```python
from build123d import *

# Parameters (mm, degrees)
F0_R     = 0.4
F0_W     = 3.627236
F0_H     = 6.562536
F0_W_2   = 7.74
F0_H_2   = 7.54
F0_W_3   = 1.741074
F0_H_3   = 3.515658
F1_DEPTH = 0.8
F2_W     = 1.5
F2_H     = 7.54
F2_W_2   = 7.74
F3_DEPTH = 3.7
F4_DEPTH = 0.6
F2_W_3   = 3.627236
F2_H_2   = 6.562536
F2_W_4   = 1.741074
F2_H_3   = 3.515658
F5_DEPTH = 1.8
F6_DEPTH = 2.5
F7_W     = 3.138918
F7_H     = 1.686543
F7_W_2   = 7.430458
F7_H_2   = 3.743672
F7_W_3   = 2.755912
F7_H_3   = 4.345508
F7_W_4   = 2.256349
F7_H_4   = 1.289181
F8_DEPTH = 1.5


with BuildPart() as f1:
    # F0 (on Top) → F1 (new body, symmetric)
    with BuildSketch(Plane.XY):
        Polygon((21.675, -8.905), (21.675, 8.905), (-21.675, 8.905), (-21.675, 3.77), (-13.935, 3.77), (-13.935, -3.77), (-21.675, -3.77), (-21.675, -8.905), align=None)
        with Locations((-19.378522, -6.999998)):
            Circle(F0_R, mode=Mode.SUBTRACT)
        with Locations((-16.578532, -6.992826)):
            Circle(F0_R, mode=Mode.SUBTRACT)
        with Locations((-13.778541, -6.985653)):
            Circle(F0_R, mode=Mode.SUBTRACT)
        with Locations((-10.97855, -6.978481)):
            Circle(F0_R, mode=Mode.SUBTRACT)
        with Locations((-8.178559, -6.971308)):
            Circle(F0_R, mode=Mode.SUBTRACT)
        with Locations((-5.378568, -6.964136)):
            Circle(F0_R, mode=Mode.SUBTRACT)
        with Locations((-2.578578, -6.956963)):
            Circle(F0_R, mode=Mode.SUBTRACT)
        with Locations((0.221413, -6.949791)):
            Circle(F0_R, mode=Mode.SUBTRACT)
        with Locations((3.021404, -6.942618)):
            Circle(F0_R, mode=Mode.SUBTRACT)
        with Locations((5.821395, -6.935446)):
            Circle(F0_R, mode=Mode.SUBTRACT)
        with Locations((8.621386, -6.928273)):
            Circle(F0_R, mode=Mode.SUBTRACT)
        with Locations((11.421377, -6.921101)):
            Circle(F0_R, mode=Mode.SUBTRACT)
        with Locations((14.221367, -6.913928)):
            Circle(F0_R, mode=Mode.SUBTRACT)
        with Locations((17.021358, -6.906755)):
            Circle(F0_R, mode=Mode.SUBTRACT)
        with Locations((19.821349, -6.899583)):
            Circle(F0_R, mode=Mode.SUBTRACT)
        Polygon((-0.115967, -0.994175), (-5.560689, -6.438898), (-11.005411, -0.994175), (-5.560689, 4.450547), align=None, mode=Mode.SUBTRACT)
        with Locations((16.957284, -2.671687)):
            Circle(F0_R, mode=Mode.SUBTRACT)
        with Locations((19.757274, -2.664514)):
            Circle(F0_R, mode=Mode.SUBTRACT)
        with Locations((16.978642, -0.005869)):
            Circle(F0_R, mode=Mode.SUBTRACT)
        with Locations((5.141591, 0)):
            Rectangle(F0_W, F0_H, mode=Mode.SUBTRACT)
        with Locations((19.778633, 0.001303)):
            Circle(F0_R, mode=Mode.SUBTRACT)
        with Locations((17, 2.659948)):
            Circle(F0_R, mode=Mode.SUBTRACT)
        with Locations((19.799991, 2.667121)):
            Circle(F0_R, mode=Mode.SUBTRACT)
        with Locations((-19.378522, 7.092626)):
            Circle(F0_R, mode=Mode.SUBTRACT)
        with Locations((-16.578532, 7.099799)):
            Circle(F0_R, mode=Mode.SUBTRACT)
        with Locations((-13.778541, 7.106971)):
            Circle(F0_R, mode=Mode.SUBTRACT)
        with Locations((-10.97855, 7.114144)):
            Circle(F0_R, mode=Mode.SUBTRACT)
        with Locations((-8.178559, 7.121316)):
            Circle(F0_R, mode=Mode.SUBTRACT)
        with Locations((-5.378568, 7.128489)):
            Circle(F0_R, mode=Mode.SUBTRACT)
        with Locations((-2.578578, 7.135661)):
            Circle(F0_R, mode=Mode.SUBTRACT)
        with Locations((0.221413, 7.142834)):
            Circle(F0_R, mode=Mode.SUBTRACT)
        with Locations((3.021404, 7.150007)):
            Circle(F0_R, mode=Mode.SUBTRACT)
        with Locations((5.821395, 7.157179)):
            Circle(F0_R, mode=Mode.SUBTRACT)
        with Locations((8.621386, 7.164352)):
            Circle(F0_R, mode=Mode.SUBTRACT)
        with Locations((11.421377, 7.171524)):
            Circle(F0_R, mode=Mode.SUBTRACT)
        with Locations((14.221367, 7.178697)):
            Circle(F0_R, mode=Mode.SUBTRACT)
        with Locations((17.021358, 7.185869)):
            Circle(F0_R, mode=Mode.SUBTRACT)
        with Locations((19.821349, 7.193042)):
            Circle(F0_R, mode=Mode.SUBTRACT)
        with Locations((-17.805, 0)):
            Rectangle(F0_W_2, F0_H_2)
        Polygon((-11.005411, -0.994175), (-5.560689, -6.438898), (-0.115967, -0.994175), (-5.560689, 4.450547), align=None)
        with Locations((5.141591, 0)):
            Rectangle(F0_W, F0_H)
        with Locations((5.141591, 0)):
            Rectangle(F0_W_3, F0_H_3, mode=Mode.SUBTRACT)
        with Locations((5.141591, 0)):
            Rectangle(F0_W_3, F0_H_3)
    extrude(amount=F1_DEPTH, both=True)

    # F2 (on face) → F3 (join)
    with BuildSketch(Plane.XY.offset(0.8)):
        with Locations((-22.425, 0)):
            Rectangle(F2_W, F2_H)
        with Locations((-17.805, 0)):
            Rectangle(F2_W_2, F2_H)
    extrude(amount=F3_DEPTH)

    # F2 (on face) → F4 (join)
    with BuildSketch(Plane.XY.offset(0.8)):
        Polygon((-5.560689, 5.444722), (-11.005411, 0), (-5.560689, -5.538898), (0, 0), align=None)
    extrude(amount=F4_DEPTH)

    # F2 (on face) → F5 (join)
    with BuildSketch(Plane.XY.offset(0.8)):
        with Locations((5.141591, 0)):
            Rectangle(F2_W_3, F2_H_2)
        with Locations((5.141591, 0)):
            Rectangle(F2_W_4, F2_H_3, mode=Mode.SUBTRACT)
    extrude(amount=F5_DEPTH)

    # F2 (on face) → F6 (join)
    with BuildSketch(Plane.XY.offset(0.8)):
        with Locations((5.141591, 0)):
            Rectangle(F2_W_4, F2_H_3)
    extrude(amount=F6_DEPTH)

    # F7 (on face) → F8 (join)
    with BuildSketch(Plane(origin=(0, 0, -0.8), x_dir=(1, 0, 0), z_dir=(0, 0, -1))):
        with Locations((-19.302629, -5.330686)):
            Rectangle(F7_W, F7_H)
        with Locations((-12.91917, 0)):
            Rectangle(F7_W_2, F7_H_2)
        with Locations((12.990596, 3.507671)):
            Rectangle(F7_W_3, F7_H_3)
        with Locations((13.02365, -1.36955)):
            Rectangle(F7_W_4, F7_H_4)
    extrude(amount=F8_DEPTH)


solid = f1.part
```
Design review of the part built by this model. Coordinates are the model's own, in mm. A direction names the side the tool comes from. Give positions to 0.01 mm unless a question says otherwise; leave off trailing zeros. Write each loop counter-clockwise with the first axis right and the second up, starting at its lowest first coordinate (ties: lowest second). Pieces come first, ordered by that corner, then holes. Notation, with made-up numbers: (19, 68.5) -> (77, 68.5) arc R30 cw to (77, 103.5) -> close; hole circle Ø11 at (-33.75, -40). An arc over 180 degrees is marked (long way). Answer in a Markdown table with one row per item.
(1) To check wall thickness, follow probe 1 along Y at (x, z) = (6, 0.5) (3 decimals); probe 2 along X at (y, z) = (-2.75, 1.25) (3 decimals); probe 3 along X at (y, z) = (4.5, -0.5) (3 decimals). State the ranges of each line that lie inside material, in increasing order.
Results:
| item | result |
|---|---|
| probe 1 | -8.905 to -7.293, -6.578 to 6.799, 7.515 to 8.905 |
| probe 2 | -23.175 to -13.935, -8.302 to -2.761, 3.328 to 6.955 |
| probe 3 | -21.675 to 21.675 |
(2) Consider section A-A (z = 2). State the section outline as (x, y) points (3 decimals).
Results:
| item | result |
|---|---|
| outline | (-23.175, -3.77) -> (-13.935, -3.77) -> (-13.935, 3.77) -> (-23.175, 3.77) -> close; (3.328, -3.281) -> (6.955, -3.281) -> (6.955, 3.281) -> (3.328, 3.281) -> close |
(3) Clearance check with flat-ended pins moving along their axes: pin 1 (0.6 mm diameter, centred on y = 1.5, z = -1.5, fed in from +X); pin 2 (0.9 mm diameter, centred on x = 5.5, z = 2, fed in from -Y); pin 3 (0.7 mm diameter, centred on y = -1, z = -1.5, fed in from -X). State where each tip first meets the part, or that it passes through.
Results:
| item | result |
|---|---|
| pin 1 | x = 14.15 |
| pin 2 | y = -3.28 |
| pin 3 | x = -16.63 |
(4) For faces 1 (the flat face through (-21.675, 0, 0)), 2 (the flat face through (6.955, 0, 2)), 3 (the flat face through (11.895, 1, -2)), list the 3-axis set-ups (+Z, -Z, +X, -X, +Y, -Y) from which the entire face can be reached by the end or side of a thin tool; tool diameter is ignored.
Results:
| item | result |
|---|---|
| face 1 | -Z, -X, +Y, -Y |
| face 2 | +Z, +X, +Y, -Y |
| face 3 | -Z, +Y |
(5) Consider section C-C (x = -7). State the section outline as (y, z) points (3 decimals), then the cut area to 3 significant figures.
Results:
| item | result |
|---|---|
| outline | (-8.905, -0.8) -> (8.905, -0.8) -> (8.905, 0.8) -> (4.005, 0.8) -> (4.005, 1.4) -> (-4.075, 1.4) -> (-4.075, 0.8) -> (-8.905, 0.8) -> close |
| area | 33.3 mm2 |
(6) Mouldability with a two-part tool opening along Y and no side actions: class faces 4 (the flat face through (11.613, -3, -2)), 5 (the cylindrical face through (-13.4, 7.23, -0.01)), 6 (the flat face through (5, 3.281, 2)), 7 (the cylindrical face through (16.704, 6.942, -0.011)) as +Y half, -Y half, draft (parallel to the pull), parting line (faces both ways), or undercut.
Results:
| item | result |
|---|---|
| face 4 | draft |
| face 5 | undercut |
| face 6 | +Y half |
| face 7 | undercut |
(7) Consider section B-B (x = -15). State the section outline as (y, z) points (3 decimals), then the cut area to 3 significant figures.
Results:
| item | result |
|---|---|
| outline | (-8.905, -0.8) -> (-1.872, -0.8) -> (-1.872, -2.3) -> (1.872, -2.3) -> (1.872, -0.8) -> (8.905, -0.8) -> (8.905, 0.8) -> (3.77, 0.8) -> (3.77, 4.5) -> (-3.77, 4.5) -> (-3.77, 0.8) -> (-8.905, 0.8) -> close |
| area | 62.0 mm2 |
